The model under review builds one solid part; all positions refer to its coordinate system, in mm. Face numbers are marked on the shaded views. A direction names the side the tool comes from. Coordinates: 2 decimals unless noted, no trailing zeros. Answer in a Markdown table with one row per item. Add a question column.
(1) Machinability: for the marked faces 1 and 2, which of the approach directions +Z, -Z, +X, -X, +Y, -Y give a long, thin tool a straight path to every point of the face, cutting with its end or side? Answer none if there is none.
(2) For P1, Ø1.1, axis at x = -7, y = -30, coming from the -Z side; P2, Ø3, axis at x = -13.5, y = -9, coming from the -Z side; P3, Ø0.5, axis at x = 7, z = 8, coming from the -Y side; P4, Ø0.8, axis at y = -30, z = 8, coming from the -X side, all flat-tipped, find the tip position at first contact; note any pin that passes through.
(3) Mouldability with a two-part tool opening along X and no side actions: class the marked faces 3, 4, 5 and 6 as +X half, -X half, draft (parallel to the pull), parting line (faces both ways), or undercut.
(4) For line 1 along Y through (x, z) = (-4, 10.5); line 2 along X through (y, z) = (26, 15); line 3 along Y through (x, z) = (-2, 13.5), list the stretches that pass through material, from the lowest coordinate up.
(5) We need section B-B on z = 13.25. Give the number of separate pieces and of enclosed holes in the cut face, plus the area to 3 significant figures.
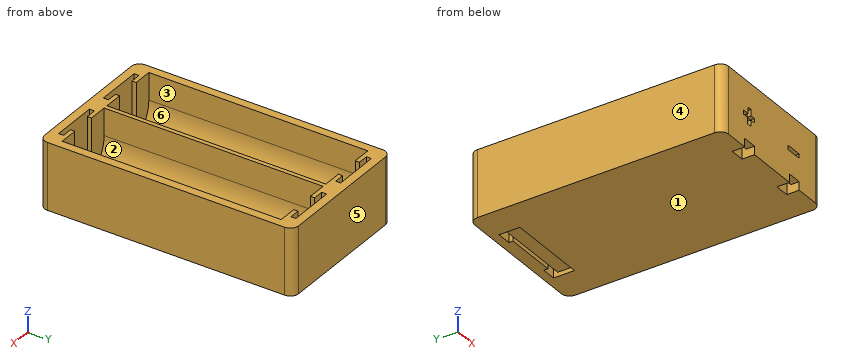
from build123d import *

# Parameters (mm, degrees)
SKETCH_W        = 35
SKETCH_H        = 61
PAD_DEPTH       = 16
SKETCH001_W     = 31
SKETCH001_H     = 57
POCKET_DEPTH    = 14
SKETCH002_W     = 1
SKETCH002_H     = 57
PAD001_DEPTH    = 14
SKETCH003_W     = 15
SKETCH003_H     = 2.2
PAD002_DEPTH    = 2
SKETCH004_W     = 3.5
SKETCH004_H     = 1
POCKET001_DEPTH = 5
SKETCH005_W     = 4.5
SKETCH005_H     = 1
PAD003_DEPTH    = 12
FILLET_R        = 2
FILLET001_R     = 7.49
SKETCH006_W     = 2
SKETCH006_H     = 1.2
PAD004_DEPTH    = 12
SKETCH007_W     = 3.5
SKETCH007_H     = 2
POCKET002_DEPTH = 2
SKETCH008_W     = 4
SKETCH008_H     = 1
POCKET003_DEPTH = 1
SKETCH009_W     = 19.5
SKETCH009_H     = 4
POCKET004_DEPTH = 1


with BuildPart() as part:
    # Sketch → Pad (new body)
    with BuildSketch(Plane.XY):
        Rectangle(SKETCH_W, SKETCH_H)
    extrude(amount=PAD_DEPTH)

    # Sketch001 (on Face6 of Pad) → Pocket (cut)
    with BuildSketch(Plane.XY.offset(16)):
        Rectangle(SKETCH001_W, SKETCH001_H)
    extrude(amount=-POCKET_DEPTH, mode=Mode.SUBTRACT)

    # Sketch002 (on Face11 of Pocket) → Pad001 (join)
    with BuildSketch(Plane.XY.offset(2)):
        Rectangle(SKETCH002_W, SKETCH002_H)
    extrude(amount=PAD001_DEPTH)

    # Sketch003 (on Face17 of Pad001) → Pad002 (join)
    with BuildSketch(Plane.XY.offset(2)):
        with Locations((8, 27.4)):
            Rectangle(SKETCH003_W, SKETCH003_H)
        with Locations((-8, 27.4)):
            Rectangle(SKETCH003_W, SKETCH003_H)
        with Locations((8, -27.4)):
            Rectangle(SKETCH003_W, SKETCH003_H)
        with Locations((-8, -27.4)):
            Rectangle(SKETCH003_W, SKETCH003_H)
    extrude(amount=PAD002_DEPTH)

    # Sketch004 (on Face22 of Pad002) → Pocket001 (cut)
    with BuildSketch(Plane.XY.offset(4)):
        with Locations((8, 28)):
            Rectangle(SKETCH004_W, SKETCH004_H)
        with Locations((-8, 28)):
            Rectangle(SKETCH004_W, SKETCH004_H)
        with Locations((8, -28)):
            Rectangle(SKETCH004_W, SKETCH004_H)
        with Locations((-8, -28)):
            Rectangle(SKETCH004_W, SKETCH004_H)
    extrude(amount=-POCKET001_DEPTH, mode=Mode.SUBTRACT)

    # Sketch005 (on Face30 of Pocket001) → Pad003 (join)
    with BuildSketch(Plane.XY.offset(4)):
        with Locations((-2.75, 26.8)):
            Rectangle(SKETCH005_W, SKETCH005_H)
        with Locations((-13.25, 26.8)):
            Rectangle(SKETCH005_W, SKETCH005_H)
        with Locations((2.75, 26.8)):
            Rectangle(SKETCH005_W, SKETCH005_H)
        with Locations((13.25, 26.8)):
            Rectangle(SKETCH005_W, SKETCH005_H)
        with Locations((13.25, -26.8)):
            Rectangle(SKETCH005_W, SKETCH005_H)
        with Locations((-13.25, -26.8)):
            Rectangle(SKETCH005_W, SKETCH005_H)
        with Locations((-2.75, -26.8)):
            Rectangle(SKETCH005_W, SKETCH005_H)
        with Locations((2.75, -26.8)):
            Rectangle(SKETCH005_W, SKETCH005_H)
    extrude(amount=PAD003_DEPTH)

    # Fillet
    fillet_edges = [part.edges().sort_by_distance(p)[0] for p in [
        (-17.5, 30.5, 8),
        (17.5, 30.5, 8),
        (17.5, -30.5, 8),
        (-17.5, -30.5, 8),
    ]]
    fillet(fillet_edges, radius=FILLET_R)

    # Fillet001
    fillet001_edges = [part.edges().sort_by_distance(p)[0] for p in [
        (-15.5, 0, 2),
        (-0.5, 0, 2),
        (0.5, 0, 2),
        (15.5, 0, 2),
    ]]
    fillet(fillet001_edges, radius=FILLET001_R)

    # Sketch006 (on Face36 of Fillet001) → Pad004 (join)
    with BuildSketch(Plane.XY.offset(4)):
        with Locations((-14.5, 27.9)):
            Rectangle(SKETCH006_W, SKETCH006_H)
        with Locations((-1.5, 27.9)):
            Rectangle(SKETCH006_W, SKETCH006_H)
        with Locations((1.5, 27.9)):
            Rectangle(SKETCH006_W, SKETCH006_H)
        with Locations((14.5, 27.9)):
            Rectangle(SKETCH006_W, SKETCH006_H)
        with Locations((14.5, -27.9)):
            Rectangle(SKETCH006_W, SKETCH006_H)
        with Locations((1.5, -27.9)):
            Rectangle(SKETCH006_W, SKETCH006_H)
        with Locations((-1.5, -27.9)):
            Rectangle(SKETCH006_W, SKETCH006_H)
        with Locations((-14.5, -27.9)):
            Rectangle(SKETCH006_W, SKETCH006_H)
    extrude(amount=PAD004_DEPTH)

    # Sketch007 (on Face2 of Fillet) → Pocket002 (cut)
    with BuildSketch(Plane(origin=(0, 0, 0), x_dir=(1, 0, 0), z_dir=(0, 0, -1))):
        with Locations((-8, 29.5)):
            Rectangle(SKETCH007_W, SKETCH007_H)
        with Locations((8, 29.5)):
            Rectangle(SKETCH007_W, SKETCH007_H)
    extrude(amount=-POCKET002_DEPTH, mode=Mode.SUBTRACT)

    # Sketch008 (on Face14 of Pocket002) → Pocket003 (cut)
    with BuildSketch(Plane.XZ.offset(30.5)):
        Polygon((-10.25, 8.5), (-8.5, 8.5), (-8.5, 10), (-7.5, 10), (-7.5, 8.5), (-6.25, 8.5), (-6.25, 7.5), (-7.5, 7.5), (-7.5, 6), (-8.75, 6), (-8.75, 7.5), (-10.25, 7.5), align=None)
        with Locations((7.75, 8)):
            Rectangle(SKETCH008_W, SKETCH008_H)
    extrude(amount=-POCKET003_DEPTH, mode=Mode.SUBTRACT)

    # Sketch009 (on Face43 of Pocket003) → Pocket004 (cut)
    with BuildSketch(Plane(origin=(0, 0, 0), x_dir=(1, 0, 0), z_dir=(0, 0, -1))):
        with Locations((0, -25.5)):
            Rectangle(SKETCH009_W, SKETCH009_H)
    extrude(amount=-POCKET004_DEPTH, mode=Mode.SUBTRACT)


solid = part.part
Outcome:
| question | item | result |
|---|---|---|
| 1 | face 1 | -Z, +X, -X, +Y, -Y |
| 1 | face 2 | +Z |
| 2 | P1 | z = 2 |
| 2 | P2 | z = 0 |
| 2 | P3 | y = -29.5 |
| 2 | P4 | x = -17.17 |
| 3 | face 3 | undercut |
| 3 | face 4 | -X half |
| 3 | face 5 | draft |
| 3 | face 6 | undercut |
| 4 | line 1 | -30.5 to -28.5, -27.3 to -26.3, 26.3 to 27.3, 28.5 to 30.5 |
| 4 | line 2 | -17.5 to -15.5, -0.5 to 0.5, 15.5 to 17.5 |
| 4 | line 3 | -30.5 to -26.3, 26.3 to 30.5 |
| 5 | separate pieces | 1 |
| 5 | enclosed holes | 2 |
| 5 | area | 477 mm² |
